```python
from build123d import *

# Parameters (mm, degrees)
ESBO_O1_R                = 3.1
RESSALTO_EXTRUS_O1_DEPTH = 7
CORTE_EXTRUS_O1_DEPTH    = 9.259539939


with BuildPart() as part:
    # Esboço1 → Ressalto-extrusão1 (new body)
    with BuildSketch(Plane(origin=(0, 0, 0), x_dir=(1, 0, 0), z_dir=(0, 1, 0))):
        with Locations(Location((0, 0, 0), (0, 0, 270))):
            Circle(ESBO_O1_R)
    extrude(amount=RESSALTO_EXTRUS_O1_DEPTH)

    # Esboço2 → Corte-extrusão1 (cut, through all)
    with BuildSketch(Plane(origin=(0, 7, 0), x_dir=(1, 0, 0), z_dir=(0, 1, 0))):
        with BuildLine():
            Line((-1.956270364, -1.48), (1.943729636, -1.48))
            ThreePointArc((1.943729636, -1.48), (2.297283026, -1.333553391), (2.443729636, -0.98))
            Line((2.443729636, -0.98), (2.443729636, 0.98))
            ThreePointArc((2.443729636, 0.98), (2.297283026, 1.333553391), (1.943729636, 1.48))
            Line((1.943729636, 1.48), (-1.956270364, 1.48))
            ThreePointArc((-1.956270364, 1.48), (-2.309823755, 1.333553391), (-2.456270364, 0.98))
            Line((-2.456270364, 0.98), (-2.456270364, -0.98))
            ThreePointArc((-2.456270364, -0.98), (-2.309823755, -1.333553391), (-1.956270364, -1.48))
        make_face()
    extrude(amount=-CORTE_EXTRUS_O1_DEPTH, mode=Mode.SUBTRACT)


solid = part.part
```
CAD build for the part. Positions are in the model's coordinates, mm. A direction names the side the tool comes from. Give positions to 0.01 mm unless a question says otherwise; leave off trailing zeros. Write each loop counter-clockwise with the first axis right and the second up, starting at its lowest first coordinate (ties: lowest second). Pieces come first, ordered by that corner, then holes. Notation, with made-up numbers: (43, -5) -> (76, -5) arc R10 ccw to (76, 3) -> close; hole circle Ø11 at (51.25, 0). An arc over 180 degrees is marked (long way). Write each question's results on one line, items separated by ' | '.
1. Cut at D-D, the plane z = 2.5. Write the cut outline in (x, y), then the cut area to 3 significant figures.
Geometry check:
outline: (-1.83, 0) -> (1.83, 0) -> (1.83, 7) -> (-1.83, 7) -> close | area: 25.7 mm²
2. Cut at B-B, the plane z = 0. Write the cut outline in (x, y).
Geometry check:
outline: (-3.1, 0) -> (-2.46, 0) -> (-2.46, 7) -> (-3.1, 7) -> close; (2.44, 0) -> (3.1, 0) -> (3.1, 7) -> (2.44, 7) -> close
3. Drop flat-ended pins along their axis: P1, Ø3, axis at x = 1, y = 5, coming from the -Z side; P2, Ø3, axis at y = 5, z = -2.5, coming from the +X side; P3, Ø3, axis at x = -2.5, y = 1.5, coming from the +Z side. Give the stop position or say it passes through.
Geometry check:
P1: z = -3.1 | P2: x = 2.93 | P3: z = 2.93
4. Cut at A-A, the plane x = 0. Write the cut outline in (y, z).
Geometry check:
outline: (0, -3.1) -> (7, -3.1) -> (7, -1.48) -> (0, -1.48) -> close; (0, 1.48) -> (7, 1.48) -> (7, 3.1) -> (0, 3.1) -> close
5. Wall check: probe 1 along X at (y, z) = (6.5, 1.25); probe 2 along Z at (x, y) = (0.25, 3.25); probe 3 along Z at (x, y) = (-1.5, 2.75). Give the ranges that are in metal, low to high. Write a range as [from, to].
Geometry check:
probe 1: [-2.84, -2.38], [2.36, 2.84] | probe 2: [-3.09, -1.48], [1.48, 3.09] | probe 3: [-2.71, -1.48], [1.48, 2.71]
6. Two-plate mould, pull along X, no slides. Class faces 1 (the cylindrical face through (0.931, 3.451, 2.957)), 2 (the flat face through (0, 4, -1.48)), 3 (the flat face through (0, 0, 2)): pulls with the +X half, pulls with the -X half, needs draft (parallel to the pull), parting line crosses it, or undercut.
Geometry check:
face 1: parting line crosses it | face 2: undercut | face 3: needs draft
7. Cut at C-C, the plane z = -1.75. Write the cut outline in (x, y).
Geometry check:
outline: (-2.56, 0) -> (2.56, 0) -> (2.56, 7) -> (-2.56, 7) -> close
8. Which spindle directions (+Z, -Z, +X, -X, +Y, -Y) get a long thin tool onto all of the face, cutting with end or side? Do faces 4 (the flat face through (2.444, 4, 0)), 5 (the flat face through (0, 7, 2)). Say none if no direction does.
Geometry check:
face 4: +Y, -Y | face 5: +Z, -Z, +X, -X, +Y
